Input: part model. Units: mm. Frame: model coordinates. Face numbers are marked on the shaded views. Give positions to 0.01 mm unless a question says otherwise; leave off trailing zeros. Loops run counter-clockwise (first coordinate to the right, second up) from the corner with the lowest first, then second, coordinate; pieces in that order, holes last. Notation, with made-up numbers: (79.5, 70) -> (103.5, 70) arc R34 ccw to (103.5, 100) -> close; hole circle Ø6 at (-0.75, 9.25). An arc over 180 degrees is marked (long way). One line per question, with ' | ' between items.
from build123d import *

# Parameters (mm, degrees)
F0_W        = 56.9857386872
F0_H        = 41.281120386
F0_R        = 10.0582455169
F1_DEPTH    = 25.4
F2_T1_DEPTH = 82.3857386872
F2_T3_DEPTH = 66.681120386
F3_T1_DEPTH = 83.114037845
F3_T3_DEPTH = 67.4094195437


# Not quite as in the source:
# - a fillet or chamfer that OpenCascade refuses, or shapes differently, is made with other operations: its cross-section is extruded or revolved along the edge and cut away or added


with BuildPart() as f1:
    # F0 (on Top) → F1 (new body)
    with BuildSketch(Plane.XY):
        with Locations((-38.084267173, -14.7667184938)):
            Rectangle(F0_W, F0_H)
        with Locations((-43.1615449488, -10.8050759882)):
            Circle(F0_R, mode=Mode.SUBTRACT)
    extrude(amount=F1_DEPTH)

    # F2: fillet of radius 5.08 on 5 edges, made by hand

    # F2_s2 → F2_t1 (cut)
    with BuildSketch(Plane.YZ.offset(-79.2771365166)):
        with BuildLine():
            ThreePointArc((5.8738416992, 20.32), (4.3859441476, 23.9121024484), (0.7938416992, 25.4))
            Line((0.7938416992, 25.4), (5.8738416992, 25.4))
            Line((5.8738416992, 25.4), (5.8738416992, 20.32))
        make_face()
        with BuildLine():
            ThreePointArc((-35.4072786868, 20.32), (-33.9193811352, 23.9121024484), (-30.3272786868, 25.4))
            Line((-30.3272786868, 25.4), (-35.4072786868, 25.4))
            Line((-35.4072786868, 25.4), (-35.4072786868, 20.32))
        make_face()
    extrude(amount=F2_T1_DEPTH, mode=Mode.SUBTRACT)

    # F2_s4 → F2_t3 (cut)
    with BuildSketch(Plane.XZ.offset(-18.5738416992)):
        with BuildLine():
            ThreePointArc((-66.5771365166, 20.32), (-65.089238965, 23.9121024484), (-61.4971365166, 25.4))
            Line((-61.4971365166, 25.4), (-66.5771365166, 25.4))
            Line((-66.5771365166, 25.4), (-66.5771365166, 20.32))
        make_face()
        with BuildLine():
            ThreePointArc((-9.5913978294, 20.32), (-11.0792953809, 23.9121024484), (-14.6713978294, 25.4))
            Line((-14.6713978294, 25.4), (-9.5913978294, 25.4))
            Line((-9.5913978294, 25.4), (-9.5913978294, 20.32))
        make_face()
    extrude(amount=F2_T3_DEPTH, mode=Mode.SUBTRACT)

    # F2_s5 → F2_t6 (revolve, cut)
    with BuildSketch(Plane.XZ.offset(10.8050759882)):
        with BuildLine():
            ThreePointArc((-33.103299432, 20.32), (-31.6154018804, 23.9121024484), (-28.023299432, 25.4))
            Line((-28.023299432, 25.4), (-33.103299432, 25.4))
            Line((-33.103299432, 25.4), (-33.103299432, 20.32))
        make_face()
    revolve(axis=Axis((-43.1615449488, -10.8050759882, 25.4), (0, 0, 1)), mode=Mode.SUBTRACT)

    # F3: chamfer of 5.08 on 5 edges, made by hand

    # F3_s2 → F3_t1 (cut)
    with BuildSketch(Plane.YZ.offset(-79.6412860954)):
        Polygon((5.8738416992, 5.08), (0.7938416992, 0), (5.8738416992, 0), align=None)
        Polygon((-30.3272786868, 0), (-35.4072786868, 5.08), (-35.4072786868, 0), align=None)
    extrude(amount=F3_T1_DEPTH, mode=Mode.SUBTRACT)

    # F3_s4 → F3_t3 (cut)
    with BuildSketch(Plane.XZ.offset(-18.9379912781)):
        Polygon((-61.4971365166, 0), (-66.5771365166, 5.08), (-66.5771365166, 0), align=None)
        Polygon((-14.6713978294, 0), (-9.5913978294, 5.08), (-9.5913978294, 0), align=None)
    extrude(amount=F3_T3_DEPTH, mode=Mode.SUBTRACT)

    # F3_s5 → F3_t6 (revolve, cut)
    with BuildSketch(Plane.XZ.offset(10.8050759882)):
        Polygon((-28.023299432, 0), (-33.103299432, 5.08), (-33.103299432, 0), align=None)
    revolve(axis=Axis((-43.1615449488, -10.8050759882, 0), (0, 0, 1)), mode=Mode.SUBTRACT)


solid = f1.part
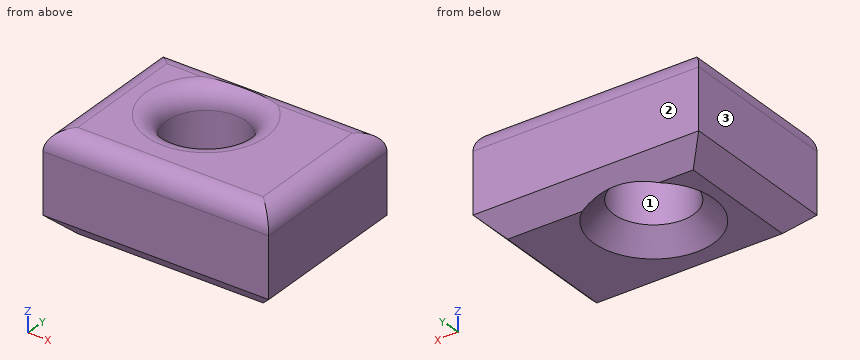
1. Section query A-A (x = -19). Output: boundary loops of the cut face in (y, z), then the cut area to 3 significant figures.
Determined:
outline: (-35.41, 5.08) -> (-30.33, 0) -> (0.79, 0) -> (5.87, 5.08) -> (5.87, 20.32) arc R5.08 ccw to (0.79, 25.4) -> (-30.33, 25.4) arc R5.08 ccw to (-35.41, 20.32) -> close | area: 1,010 mm2
2. Pull-direction query (X, two-part tool) for the marked faces 1, 2 and 3; classes: pulls with the +X half, pulls with the -X half, needs draft (parallel to the pull), parting line crosses it, or undercut.
Determined:
face 1: undercut | face 2: needs draft | face 3: pulls with the -X half
3. Section query B-B (y = -27.5). Output: boundary loops of the cut face in (x, z), then the cut area to 3 significant figures.
Determined:
outline: (-66.58, 5.08) -> (-61.5, 0) -> (-14.67, 0) -> (-9.59, 5.08) -> (-9.59, 20.32) arc R5.08 ccw to (-14.67, 25.4) -> (-61.5, 25.4) arc R5.08 ccw to (-66.58, 20.32) -> close | area: 1,410 mm2
4. Ray query, line 1 along X through (y, z) = (-10.5, 8.5); line 2 along Y through (x, z) = (-39.5, 21.25); line 3 along Y through (x, z) = (-45, 24.75). Return the intervals inside material, ascending. Write a range as from..to.
Determined:
line 1: x = -66.58..-53.22, -33.11..-9.59 | line 2: y = -35.32..-20.27, -1.34..5.79 | line 3: y = -32.81..-23.32, 1.71..3.28
5. Pin query (flat end, axial travel): P1, Ø23, axis at x = -43.16, y = -10.81, coming from the +Z side. Return the tip coordinate at first contact, or that it passes through.
Determined:
P1: stops at z = 23.87
6. Section query C-C (z = 7.25). Output: boundary loops of the cut face in (x, y), then the cut area to 3 significant figures.
Determined:
outline: (-66.58, -35.41) -> (-9.59, -35.41) -> (-9.59, 5.87) -> (-66.58, 5.87) -> close; hole circle Ø20.12 at (-43.16, -10.81) | area: 2,030 mm2
